Check sheet for the modelled part. Datum: model origin and axes. Units: mm. A direction names the side the tool comes from. Round coordinates to 2 decimals unless told otherwise and drop trailing zeros. Loops run counter-clockwise (first coordinate to the right, second up) from the corner with the lowest first, then second, coordinate; pieces in that order, holes last. Notation, with made-up numbers: (55, 17.25) - (85, 17.25) arc R22 ccw to (85, 24.25) - close; hole circle Ø6 at (84, 35.25). An arc over 180 degrees is marked (long way). Return JSON: item names as keys, results as strings.
Autodesk Inventor part; units mm, degrees
ref_plane "РабПлоскость1" through (0, 2.5, 0) normal (0, -1, 0) x (1, 0, 0)
ref_plane "YZ Plane" through (0, 0, 0) normal (1, 0, 0) x (0, 1, 0)
ref_plane "XZ Plane" through (0, 0, 0) normal (0, 1, 0) x (-1, 0, 0)
sketch "Эскиз1" plane through (0, 0, 0) normal (0, 1, 0) x (-1, 0, 0)
  circle A0 centre (0, 0) radius 52.5
  line L0 (89.6506, 0) -> (-102.8587, 0)
  line L1 (-27, -7.5) -> (27, -7.5)
  line L2 (30, -4.5) -> (30, 4.5)
  line L3 (27, 7.5) -> (-27, 7.5)
  line L4 (-30, 4.5) -> (-30, -4.5)
  line L5 (-30, -7.5) -> (30, 7.5) construction
  line L6 (30, -7.5) -> (-30, 7.5) construction
  arc A1 (30, 4.5) -> (27, 7.5) centre (27, 4.5) ccw
  arc A2 (27, -7.5) -> (30, -4.5) centre (27, -4.5) ccw
  arc A3 (-27, 7.5) -> (-30, 4.5) centre (-27, 4.5) ccw
  arc A4 (-30, -4.5) -> (-27, -7.5) centre (-27, -4.5) ccw
  line L7 (33, -12) -> (-33, -12)
  line L8 (-35, -10) -> (-35, 10)
  line L9 (-33, 12) -> (33, 12)
  line L10 (35, 10) -> (35, -10)
  line L11 (35, -12) -> (-32.3514, 11.0919) construction
  line L12 (-35, -12) -> (35, 12) construction
  arc A5 (-33, 12) -> (-35, 10) centre (-33, 10) ccw
  arc A6 (-35, -10) -> (-33, -12) centre (-33, -10) ccw
  arc A7 (33, -12) -> (35, -10) centre (33, -10) ccw
  arc A8 (35, 10) -> (33, 12) centre (33, 10) ccw
  point P0 (-35, 12)
  dimension "d0" = 105
  dimension "d1" = 60
  dimension "d2" = 15
  dimension "d3" = 3
  dimension "d4" = 3
  dimension "d13" = 70
  dimension "d14" = 24
  dimension "d15" = 2
extrude "Выдавливание1" add sketch "Эскиз1" along normal blind 5 contours L0 L10 A8 L9 A5 L8 A0 | A0 L0 L8 A6 L7 A7 L10 | L10 A7 L7 A6 L8 L0 L4 A4 L1 A2 L2 | L0 L2 A1 L3 A3 L4 L8 A5 L9 A8 L10
chamfer "Фаска1" distance 3 angle 45 8 edges at (0, 5, 7.5) (-29.1213, 5, 6.6213) (-30, 5, 0) (-29.1213, 5, -6.6213) (0, 5, -7.5) (29.1213, 5, -6.6213) (30, 5, 0) (29.1213, 5, 6.6213)
chamfer "Фаска2" distance 1 angle 45 1 edges at (52.5, 5, 0)
extrude "Выдавливание2" cut sketch "Эскиз1" along normal blind 1.5 contours L10 A7 L7 A6 L8 L0 L4 A4 L1 A2 L2 | L0 L2 A1 L3 A3 L4 L8 A5 L9 A8 L10 | L2 A2 L1 A4 L4 L0 | L0 L4 A3 L3 A1 L2
ref_plane "РабПлоскость1" through (0, 2.5, 0) normal (0, -1, 0) x (1, 0, 0)
properties part number "фланец2" material "Термопластическая смола"
Q1. Scan lines: probe 1 along Z at (x, y) = (0.5, 0.35); probe 2 along Z at (x, y) = (-11, 4.3); probe 3 along X at (y, z) = (4, -4). Record each from-to range of solid material in increasing order. Write a range as [from, to].
Answer key:
{"probe 1": "z = [-52.5, -12], [12, 52.5]", "probe 2": "z = [-51.03, -9.8], [9.8, 51.03]", "probe 3": "x = [-52.35, -32], [32, 52.35]"}
Q2. Draft check along Z on faces 5 (the face through (-50.076, 1.972, -15.77)), 6 (the face through (-29.994, 3.188, 7.428)), 7 (the face through (29.14, 1.75, 6.6)), 8 (the face through (1, 5, -11)). Enter one of: released by +Z, released by -Z, zero draft, split by the parting line, or undercut.
Answer key:
{"face 5": "split by the parting line", "face 6": "undercut", "face 7": "undercut", "face 8": "zero draft"}
Q3. Depth check by flat-ended pin: P1, Ø1.2, axis at x = -3, y = 0.5, coming from the +Z side; P2, Ø1.2, axis at x = -15.5, y = 0.5, coming from the -Z side; P3, Ø3, axis at x = -1, y = 1.5, coming from the +Z side. Enter the tip coordinate at first touch or a pass-through.
Answer key:
{"P1": "stops at z = 52.45", "P2": "stops at z = -50.34", "P3": "stops at z = 52.5"}
Q4. Tool access check on faces 1 (the face through (0.4, 3.5, -9)), 2 (the face through (0, 1.5, 8)), 3 (the face through (-29.1, 1.75, 6.64)), 4 (the face through (0.7, 0, 12.4)). Record the directions out of +Z, -Z, +X, -X, +Y, -Y that give a thin tool (end or side, any length) a straight path to the whole face; none if there is none.
Answer key:
{"face 1": "+Y", "face 2": "-Y", "face 3": "+Y, -Y", "face 4": "+Z, -Z, +X, -X, -Y"}
Q5. Sectioned sample at A-A (x = 0). Enter the section's corners in (y, z), plus the area to 4 significant figures.
Answer key:
{"outline": "(0, -52.5) - (4, -52.5) - (5, -51.5) - (5, -10.5) - (2, -7.5) - (1.5, -7.5) - (1.5, -12) - (0, -12) - close; (0, 12) - (1.5, 12) - (1.5, 7.5) - (2, 7.5) - (5, 10.5) - (5, 51.5) - (4, 52.5) - (0, 52.5) - close", "area": "426.5 mm²"}
